Source: CAD feature listing. Evaluate the final solid. Frame: model axes, mm. A direction names the side the tool comes from. Coordinates: 2 decimals unless noted, no trailing zeros. Write each loop counter-clockwise with the first axis right and the second up, starting at its lowest first coordinate (ties: lowest second). Pieces come first, ordered by that corner, then holes. Notation, with made-up numbers: (-9.75, 65.25) -> (49.25, 65.25) arc R19 cw to (49.25, 92.25) -> close; hole circle Ø7 at (41, 58). An arc over 180 degrees is marked (long way). One line per item, written item: value. Start each with the question number.
1. First-contact query: P1, Ø1.8, axis at x = -1.5, y = 23, coming from the -Z side; P2, Ø1.8, axis at x = -0.5, z = -10, coming from the -Y side; P3, Ø2, axis at x = -0.5, z = -8, coming from the +Y side. Flat tips, straight axial feed; report the tip coordinate or a pass-through.
2. Section query D-D, the plane z = -11. Output: boundary loops of the cut face in (x, y).
3. Section query A-A, the plane x = 1.35. Output: boundary loops of the cut face in (y, z).
4. Access query for faces 1 (the flat face through (0, 13, 3)), 2 (the flat face through (0, 11, -10)), 3 (the flat face through (0, 21, -3)), 4 (the flat face through (1.969, 13, -10)), 5 (the flat face through (2.5, 13, 0)). Directions: +Z, -Z, +X, -X, +Y, -Y. A direction counts if a zero-diameter tool reaches every point of the face in a straight line with its end or side. Return the directions, or none.
5. Section query C-C, the plane y = 9. Output: boundary loops of the cut face in (x, z).
6. Mould query, pull axis X, two halves, no side actions, for faces 6 (the flat face through (2.969, 13, -3)), 7 (the flat face through (2.2, 12.8, -2.526)), 8 (the flat face through (-2.7, 0, 0)). Classes: released by +X, released by -X, zero draft, split by the parting line, or undercut.
7. Section query B-B, the plane z = -1.75. Output: boundary loops of the cut face in (x, y).
8. Line query: line 1 (Y direction, x = 1.45, z = -6.75); line 2 (Z direction, x = 0.5, y = 6); line 3 (X direction, y = 14.25, z = -1). Output: solid intervals per line, ascending.
from build123d import *

# Parameters (mm, degrees)
SKETCH1_W           = 5.93875838
SKETCH1_H           = 6
SKETCH1_W_2         = 5
SKETCH1_H_2         = 5.051560964
BOSS_EXTRUDE1_DEPTH = 26
SKETCH4_W           = 5.93875838
SKETCH4_H           = 5
BOSS_EXTRUDE2_DEPTH = 14.5
SKETCH5_W           = 4
SKETCH5_H           = 4
CUT_EXTRUDE1_DEPTH  = 14.974219518


with BuildPart() as part:
    # Sketch1 → Boss-Extrude1 (new body)
    with BuildSketch(Plane(origin=(0, 0, 0), x_dir=(1, 0, 0), z_dir=(0, 1, 0))):
        Rectangle(SKETCH1_W, SKETCH1_H)
        Rectangle(SKETCH1_W_2, SKETCH1_H_2, mode=Mode.SUBTRACT)
    extrude(amount=BOSS_EXTRUDE1_DEPTH)

    # Sketch4 → Boss-Extrude2 (add)
    with BuildSketch(Plane(origin=(0, 0, -3), x_dir=(-1, 0, 0), z_dir=(0, 0, -1))):
        with Locations((0, 13.5)):
            Rectangle(SKETCH4_W, SKETCH4_H)
    extrude(amount=BOSS_EXTRUDE2_DEPTH)

    # Sketch5 → Cut-Extrude1 (cut)
    with BuildSketch(Plane(origin=(0, 0, -17.5), x_dir=(-1, 0, 0), z_dir=(0, 0, -1))):
        with Locations((0.03062081, 13.5)):
            Rectangle(SKETCH5_W, SKETCH5_H)
    extrude(amount=-CUT_EXTRUDE1_DEPTH, mode=Mode.SUBTRACT)


solid = part.part
Computed values:
1. P1: stops at z = -3
1. P2: stops at y = 11
1. P3: stops at y = 16
2. outline: (-2.97, 11) -> (2.97, 11) -> (2.97, 16) -> (-2.97, 16) -> close; hole (-2.03, 11.5) -> (1.97, 11.5) -> (1.97, 15.5) -> (-2.03, 15.5) -> close
3. outline: (0, -3) -> (11, -3) -> (11, -17.5) -> (11.5, -17.5) -> (11.5, -2.53) -> (0, -2.53) -> close; (0, 2.53) -> (26, 2.53) -> (26, 3) -> (0, 3) -> close; (15.5, -17.5) -> (16, -17.5) -> (16, -3) -> (26, -3) -> (26, -2.53) -> (15.5, -2.53) -> close
4. face 1: +Z, +X, -X, +Y, -Y
4. face 2: -Z, +X, -X, -Y
4. face 3: -Z, +X, -X, +Y
4. face 4: -Z
4. face 5: +Y, -Y
5. outline: (-2.97, -3) -> (2.97, -3) -> (2.97, 3) -> (-2.97, 3) -> close; hole (-2.5, -2.53) -> (2.5, -2.53) -> (2.5, 2.53) -> (-2.5, 2.53) -> close
6. face 6: released by +X
6. face 7: undercut
6. face 8: zero draft
7. outline: (-2.97, 0) -> (-2.5, 0) -> (-2.5, 26) -> (-2.97, 26) -> close; (2.5, 0) -> (2.97, 0) -> (2.97, 26) -> (2.5, 26) -> close
8. line 1: y = 11 to 11.5, 15.5 to 16
8. line 2: z = -3 to -2.53, 2.53 to 3
8. line 3: x = -2.97 to -2.5, 2.5 to 2.97
